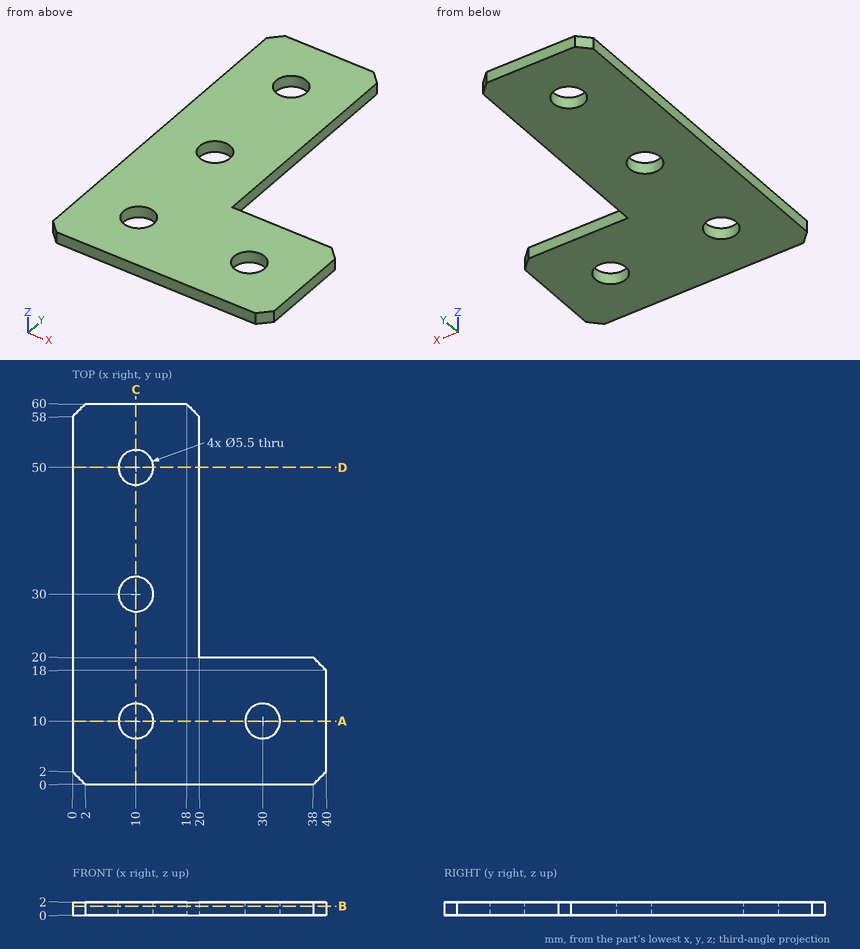
Geometry: see drawing. Coordinates: mm, zero at the bounding-box minimum. Give positions to 0.01 mm unless a question says otherwise; leave off trailing zeros. Loops run counter-clockwise (first coordinate to the right, second up) from the corner with the lowest first, then second, coordinate; pieces in that order, holes last. Notation, with made-up numbers: (-26, 5.25) -> (28, 5.25) arc R15 cw to (28, 23.25) -> close; hole circle Ø5 at (-3.75, 33.5). An arc over 180 degrees is marked (long way). Answer as a JSON object with one key per item and string values. Group by question number.
Item 1: Line query: probe 1 along Y at (x, z) = (10, 1.2); probe 2 along X at (y, z) = (10, 1.3); probe 3 along X at (y, z) = (8.5, 0.3). Output: solid intervals per line, ascending.
Item 2: Cut plane A-A, the plane y = 10. Return the cut outline in (x, z).
Item 3: Cut plane C-C, the plane x = 10. Return the cut outline in (y, z), and give its area (3 significant figures).
Item 4: Cut plane D-D, the plane y = 50. Return the cut outline in (x, z).
Item 5: Cut plane B-B, the plane z = 1.4. Return the cut outline in (x, y).
Item 6: Pin query (flat end, axial travel): P1, Ø9, axis at x = 30, y = 10, coming from the -Z side. Return the tip coordinate at first contact, or that it passes through.
Checks:
{
 "1": {"probe 1": "y = 0 to 7.25, 12.75 to 27.25, 32.75 to 47.25, 52.75 to 60", "probe 2": "x = 0 to 7.25, 12.75 to 27.25, 32.75 to 40", "probe 3": "x = 0 to 7.7, 12.3 to 27.7, 32.3 to 40"},
 "2": {"outline": "(0, 0) -> (7.25, 0) -> (7.25, 2) -> (0, 2) -> close; (12.75, 0) -> (27.25, 0) -> (27.25, 2) -> (12.75, 2) -> close; (32.75, 0) -> (40, 0) -> (40, 2) -> (32.75, 2) -> close"},
 "3": {"outline": "(0, 0) -> (7.25, 0) -> (7.25, 2) -> (0, 2) -> close; (12.75, 0) -> (27.25, 0) -> (27.25, 2) -> (12.75, 2) -> close; (32.75, 0) -> (47.25, 0) -> (47.25, 2) -> (32.75, 2) -> close; (52.75, 0) -> (60, 0) -> (60, 2) -> (52.75, 2) -> close", "area": "87.0 mm²"},
 "4": {"outline": "(0, 0) -> (7.25, 0) -> (7.25, 2) -> (0, 2) -> close; (12.75, 0) -> (20, 0) -> (20, 2) -> (12.75, 2) -> close"},
 "5": {"outline": "(0, 2) -> (2, 0) -> (38, 0) -> (40, 2) -> (40, 18) -> (38, 20) -> (20, 20) -> (20, 58) -> (18, 60) -> (2, 60) -> (0, 58) -> close; hole circle Ø5.5 at (10, 10); hole circle Ø5.5 at (10, 30); hole circle Ø5.5 at (10, 50); hole circle Ø5.5 at (30, 10)"},
 "6": {"P1": "stops at z = 0"}
}
